The figure shows three views and two pictorial views of one solid part (mm, origin at its lowest corner). Answer the questions. Coordinates: 2 decimals unless noted, no trailing zeros. Order: outer loops, then holes, each group sorted by start corner. A loop starts at its lowest first (then second) coordinate and runs counter-clockwise, first axis right, second up. Notation, with made-up numbers: M 47,-4.75 L 84,-4.75 A15 cw 84,0.25 Z; hole C 19,6.25 d7. An arc over 180 degrees is marked long. Use a Markdown table: item, result.
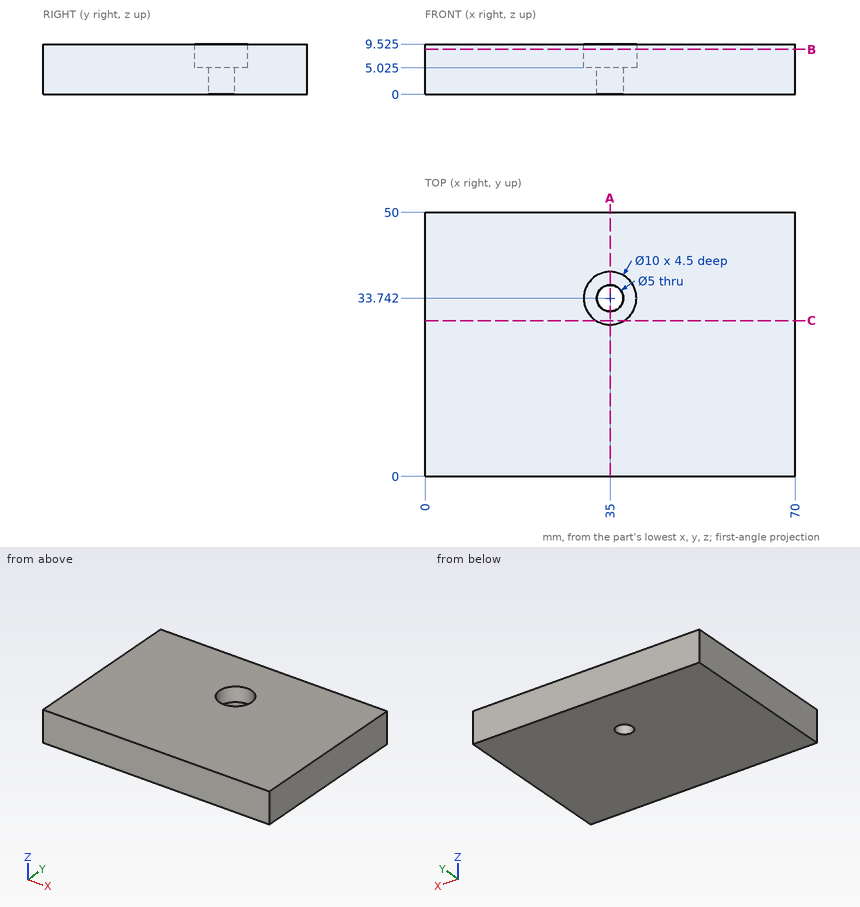
1. Section C-C on y = 29.5 is taken. Determine the outline of the cut face in (x, z) (1 decimal), then the cut area to 3 significant figures.
Answers below:
| item | result |
|---|---|
| outline | M 0,0 L 70,0 L 70,9.5 L 37.6,9.5 L 37.6,5 L 32.4,5 L 32.4,9.5 L 0,9.5 Z |
| area | 643 mm² |
2. Section A-A on x = 35 is taken. Determine the outline of the cut face in (y, z) (1 decimal).
Answers below:
| item | result |
|---|---|
| outline | M 0,0 L 31.2,0 L 31.2,5 L 28.7,5 L 28.7,9.5 L 0,9.5 Z; M 36.2,0 L 50,0 L 50,9.5 L 38.7,9.5 L 38.7,5 L 36.2,5 Z |
3. Find the intervals of material crossed by probe 1 along Y at (x, z) = (35, 6.25); probe 2 along Y at (x, z) = (35, 3.15); probe 3 along X at (y, z) = (33, 1), in increasing order.
Answers below:
| item | result |
|---|---|
| probe 1 | 0 to 28.74, 38.74 to 50 |
| probe 2 | 0 to 31.24, 36.24 to 50 |
| probe 3 | 0 to 32.61, 37.39 to 70 |
4. Section B-B on z = 8.5 is taken. Determine the outline of the cut face in (x, y), then the cut area to 3 significant figures.
Answers below:
| item | result |
|---|---|
| outline | M 0,0 L 70,0 L 70,50 L 0,50 Z; hole C 35,33.74 d10 |
| area | 3,420 mm² |
5. A flat-ended cylindrical pin translates along its axis: P1, Ø6, axis at x = 35, y = 33.74, coming from the +Z side (3 decimals). Find the tip coordinate at first contact, or state that the pin passes through.
Answers below:
| item | result |
|---|---|
| P1 | z = 5.025 |
